Answer from the drawing. Dimensions are ordinates in mm from the lowest x, y and z of the part. A direction names the side the tool comes from. Coordinates: 2 decimals unless noted, no trailing zeros. Write each loop counter-clockwise with the first axis right and the second up, starting at its lowest first coordinate (ties: lowest second). Pieces come first, ordered by that corner, then holes. Notation, with made-up numbers: (30, 11) - (71, 11) arc R22 ccw to (71, 46) - close; hole circle Ø3 at (-36.5, 6.5). An arc over 180 degrees is marked (long way). Use a Markdown table: item, result.
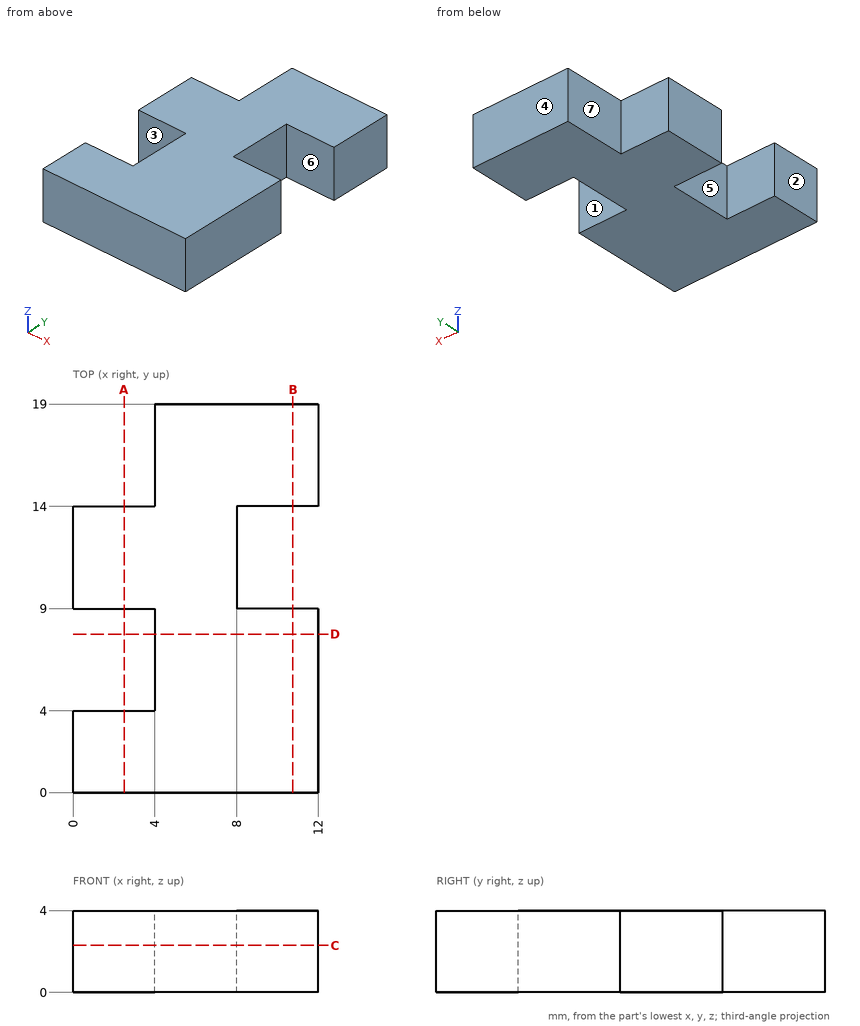
(1) A cutting plane is placed at B-B, the plane x = 10.75. Write down the section's boundary in (y, z), and give its area (3 significant figures).
Report:
| item | result |
|---|---|
| outline | (0, 0) - (9, 0) - (9, 4) - (0, 4) - close; (14, 0) - (19, 0) - (19, 4) - (14, 4) - close |
| area | 56.0 mm² |
(2) The mould has two halves that part along Y. Classify the marked faces 1, 2, 3 and 4: pulls with the +Y half, pulls with the -Y half, needs draft (parallel to the pull), parting line crosses it, or undercut.
Report:
| item | result |
|---|---|
| face 1 | undercut |
| face 2 | needs draft |
| face 3 | undercut |
| face 4 | pulls with the +Y half |
(3) Straight lines are drawn through the part: L1, parallel to Y at x = 3.75, z = 3.4; L2, parallel to X at y = 17.75, z = 2.55; L3, parallel to Y at x = 10, z = 1.05. For each, find the intervals that lie inside material, in ascending order.
Report:
| item | result |
|---|---|
| L1 | y = 0 to 4, 9 to 14 |
| L2 | x = 4 to 12 |
| L3 | y = 0 to 9, 14 to 19 |
(4) A cutting plane is placed at A-A, the plane x = 2.5. Write down the section's boundary in (y, z).
Report:
| item | result |
|---|---|
| outline | (0, 0) - (4, 0) - (4, 4) - (0, 4) - close; (9, 0) - (14, 0) - (14, 4) - (9, 4) - close |
(5) For the marked faces 5, 6 and 7, determine the directions among +Z, -Z, +X, -X, +Y, -Y from which every point of the face is accessible in a straight line to the end or side of a thin tool.
Report:
| item | result |
|---|---|
| face 5 | +Z, -Z, -X |
| face 6 | +Z, -Z, +X |
| face 7 | +Z, -Z, -X, +Y |
(6) A cutting plane is placed at D-D, the plane y = 7.75. Write down the section's boundary in (x, z).
Report:
| item | result |
|---|---|
| outline | (4, 0) - (12, 0) - (12, 4) - (4, 4) - close |
(7) Each of these flat-tipped pins is pushed along its axis until it touches: P1, Ø1.2, axis at x = 1, z = 2.5, coming from the +Y side; P2, Ø2, axis at y = 7.5, z = 2.5, coming from the -X side. Where does it stop, or does it pass through?
Report:
| item | result |
|---|---|
| P1 | stops at y = 14 |
| P2 | stops at x = 4 |
(8) A cutting plane is placed at C-C, the plane z = 2.3. Write down the section's boundary in (x, y), and give its area (3 significant figures).
Report:
| item | result |
|---|---|
| outline | (0, 0) - (12, 0) - (12, 9) - (8, 9) - (8, 14) - (12, 14) - (12, 19) - (4, 19) - (4, 14) - (0, 14) - (0, 9) - (4, 9) - (4, 4) - (0, 4) - close |
| area | 168 mm² |
